from build123d import *

# Parameters (mm, degrees)
S01_BEARING_BARREL_R                             = 22
F_01_BEARING_BARREL_DEPTH                        = 21
F_02_TORQUE_ARM_1_DEPTH                          = 10
F_03_TORQUE_ARM_2_DEPTH                          = 10
F_04_TORQUE_ARM_3_DEPTH                          = 10
F_05_WHEEL_ARM_ROOT_TO_ROUNDED_ELBOW_DEPTH       = 10
F_06_LONG_DROPPED_WHEEL_ARM_DEPTH                = 10
F_07_BROAD_CAM_FOLLOWER_MOUNTING_LUG_DEPTH       = 10
F_08_START                                       = -1
S08_BEARING_THROUGH_RELIEF_R                     = 12
F_08_BEARING_THROUGH_RELIEF_DEPTH                = 23
F_09_START                                       = -0.1
S09_INBOARD_6001_SEAT_R                          = 14.1
F_09_INBOARD_6001_SEAT_DEPTH                     = 8.2
F_10_START                                       = 12.9
S10_OUTBOARD_6001_SEAT_R                         = 14.1
F_10_OUTBOARD_6001_SEAT_DEPTH                    = 8.2
F_11_START                                       = -1
S11_KEEPER_SCREWS_R                              = 1.7
F_11_KEEPER_SCREWS_DEPTH                         = 23
F_12_START                                       = -1
S12_TORQUE_PIN_RETAINING_STEMS_R                 = 3.25
F_12_TORQUE_PIN_RETAINING_STEMS_DEPTH            = 12
F_19_START                                       = -1
S19_THROUGH_BORE_FOR_STEEL_FOLLOWER_BU_R         = 5.1
F_19_THROUGH_BORE_FOR_STEEL_FOLLOWER_BUS_DEPTH   = 12
F_20_START                                       = -0.1
S20_FLUSH_SEAT_FOR_BUSH_FLANGE_R                 = 7.6
F_20_FLUSH_SEAT_FOR_BUSH_FLANGE_DEPTH            = 2.1
FLAT_MOTOR_MOUNTING_PAD_LAYOUT_R                 = 21
FLAT_MOTOR_MOUNTING_PAD_DEPTH                    = 10
R4_BLENDS_FROM_ARM_INTO_MOTOR_PAD_R              = 4
F_28_START                                       = 10.12
F_28_X_14_CLOSED_THROUGH_SLOT_FOR_MOTOR_OU_DEPTH = 10.24
SIX_START                                        = 10.12
SIX_CLEARANCE_HOLES_FROM_JOHNSON_MOT_2_R         = 1.65
SIX_CLEARANCE_HOLES_FROM_JOHNSON_MOTOR_F_DEPTH   = 10.24
F_01_START                                       = -0.1
S01_PRINTED_DRIVE_PIN_PILOT_BORES_R              = 4.1
F_01_PRINTED_DRIVE_PIN_PILOT_BORES_DEPTH         = 10.2
F_02_START                                       = -0.1
S02_FLUSH_SEATS_FOR_DRIVE_PIN_SHOULDER_R         = 5.4
F_02_FLUSH_SEATS_FOR_DRIVE_PIN_SHOULDERS_DEPTH   = 2.1


with BuildPart() as part:
    # S01 - Bearing barrel → 01 - Bearing barrel (new body)
    with BuildSketch(Plane.XY):
        with Locations(Location((0, 0, 0), (0, 0, 180))):
            Circle(S01_BEARING_BARREL_R)
    extrude(amount=F_01_BEARING_BARREL_DEPTH)

    # S02 - Torque arm 1 → 02 - Torque arm 1 (add)
    with BuildSketch(Plane.XY):
        with BuildLine():
            Line((0, 8), (36, 8))
            ThreePointArc((36, 8), (44, 0), (36, -8))
            Line((36, -8), (0, -8))
            ThreePointArc((0, -8), (-8, 0), (0, 8))
        make_face()
    extrude(amount=F_02_TORQUE_ARM_1_DEPTH)

    # S03 - Torque arm 2 → 03 - Torque arm 2 (add)
    with BuildSketch(Plane.XY):
        with BuildLine():
            Line((-6.92820323, -4), (-24.92820323, 27.176914536))
            ThreePointArc((-24.92820323, 27.176914536), (-22, 38.105117767), (-11.07179677, 35.176914536))
            Line((-11.07179677, 35.176914536), (6.92820323, 4))
            ThreePointArc((6.92820323, 4), (4, -6.92820323), (-6.92820323, -4))
        make_face()
    extrude(amount=F_03_TORQUE_ARM_2_DEPTH)

    # S04 - Torque arm 3 → 04 - Torque arm 3 (add)
    with BuildSketch(Plane.XY):
        with BuildLine():
            Line((6.92820323, -4), (-11.07179677, -35.176914536))
            ThreePointArc((-11.07179677, -35.176914536), (-22, -38.105117767), (-24.92820323, -27.176914536))
            Line((-24.92820323, -27.176914536), (-6.92820323, 4))
            ThreePointArc((-6.92820323, 4), (4, 6.92820323), (6.92820323, -4))
        make_face()
    extrude(amount=F_04_TORQUE_ARM_3_DEPTH)

    # S05 - Wheel arm root to rounded elbow → 05 - Wheel arm root to rounded elbow (add)
    with BuildSketch(Plane.XY):
        with BuildLine():
            Line((0.890943823, 12.969434032), (67.022341031, 8.426494092))
            ThreePointArc((67.022341031, 8.426494092), (79.10083124, -5.433883763), (65.240453385, -17.512373972))
            Line((65.240453385, -17.512373972), (-0.890943823, -12.969434032))
            ThreePointArc((-0.890943823, -12.969434032), (-12.969434032, 0.890943823), (0.890943823, 12.969434032))
        make_face()
    extrude(amount=F_05_WHEEL_ARM_ROOT_TO_ROUNDED_ELBOW_DEPTH)

    # S06 - Long dropped wheel arm → 06 - Long dropped wheel arm (add)
    with BuildSketch(Plane.XY):
        with BuildLine():
            Line((76.528125799, 1.449391376), (116.886494349, -68.572605409))
            ThreePointArc((116.886494349, -68.572605409), (112.482097074, -84.961665317), (96.093037167, -80.557268042))
            Line((96.093037167, -80.557268042), (55.734668617, -10.535271257))
            ThreePointArc((55.734668617, -10.535271257), (60.139065892, 5.853788651), (76.528125799, 1.449391376))
        make_face()
    extrude(amount=F_06_LONG_DROPPED_WHEEL_ARM_DEPTH)

    # S07 - Broad cam follower mounting lug → 07 - Broad cam follower mounting lug (add)
    with BuildSketch(Plane.XY):
        with BuildLine():
            Line((6.53566842, 10.064046815), (57.694573065, -23.158934321))
            ThreePointArc((57.694573065, -23.158934321), (61.22295146, -39.758649556), (44.623236224, -43.287027951))
            Line((44.623236224, -43.287027951), (-6.53566842, -10.064046815))
            ThreePointArc((-6.53566842, -10.064046815), (-10.064046815, 6.53566842), (6.53566842, 10.064046815))
        make_face()
    extrude(amount=F_07_BROAD_CAM_FOLLOWER_MOUNTING_LUG_DEPTH)

    # S08 - Bearing through relief → 08 - Bearing through relief (cut)
    with BuildSketch(Plane.XY.offset(F_08_START)):
        Circle(S08_BEARING_THROUGH_RELIEF_R)
    extrude(amount=F_08_BEARING_THROUGH_RELIEF_DEPTH, mode=Mode.SUBTRACT)

    # S09 - Inboard 6001 seat → 09 - Inboard 6001 seat (cut)
    with BuildSketch(Plane.XY.offset(F_09_START)):
        Circle(S09_INBOARD_6001_SEAT_R)
    extrude(amount=F_09_INBOARD_6001_SEAT_DEPTH, mode=Mode.SUBTRACT)

    # S10 - Outboard 6001 seat → 10 - Outboard 6001 seat (cut)
    with BuildSketch(Plane.XY.offset(F_10_START)):
        Circle(S10_OUTBOARD_6001_SEAT_R)
    extrude(amount=F_10_OUTBOARD_6001_SEAT_DEPTH, mode=Mode.SUBTRACT)

    # S11 - Keeper screws → 11 - Keeper screws (cut)
    with BuildSketch(Plane.XY.offset(F_11_START)):
        with Locations((0, 18.25)):
            Circle(S11_KEEPER_SCREWS_R)
        with Locations((-15.804963619, -9.125)):
            Circle(S11_KEEPER_SCREWS_R)
        with Locations((15.804963619, -9.125)):
            Circle(S11_KEEPER_SCREWS_R)
    extrude(amount=F_11_KEEPER_SCREWS_DEPTH, mode=Mode.SUBTRACT)

    # S12 - Torque pin retaining stems → 12 - Torque pin retaining stems (cut)
    with BuildSketch(Plane.XY.offset(F_12_START)):
        with Locations(Location((36, 0, 0), (0, 0, 180))):
            Circle(S12_TORQUE_PIN_RETAINING_STEMS_R)
        with Locations(Location((-18, 31.176914536, 0), (0, 0, 180))):
            Circle(S12_TORQUE_PIN_RETAINING_STEMS_R)
        with Locations(Location((-18, -31.176914536, 0), (0, 0, 180))):
            Circle(S12_TORQUE_PIN_RETAINING_STEMS_R)
    extrude(amount=F_12_TORQUE_PIN_RETAINING_STEMS_DEPTH, mode=Mode.SUBTRACT)

    # S19 - Through bore for steel follower bu → 19 - Through bore for steel follower bus (cut)
    with BuildSketch(Plane.XY.offset(F_19_START)):
        with Locations(Location((51.158904645, -33.222981136, 0), (0, 0, 180))):
            Circle(S19_THROUGH_BORE_FOR_STEEL_FOLLOWER_BU_R)
    extrude(amount=F_19_THROUGH_BORE_FOR_STEEL_FOLLOWER_BUS_DEPTH, mode=Mode.SUBTRACT)

    # S20 - Flush seat for bush flange → 20 - Flush seat for bush flange (cut)
    with BuildSketch(Plane.XY.offset(F_20_START)):
        with Locations((51.158904645, -33.222981136)):
            Circle(S20_FLUSH_SEAT_FOR_BUSH_FLANGE_R)
    extrude(amount=F_20_FLUSH_SEAT_FOR_BUSH_FLANGE_DEPTH, mode=Mode.SUBTRACT)

    # Flat motor mounting pad layout → Flat motor mounting pad (add)
    with BuildSketch(Plane.XY):
        with Locations((106.780015642, -75.748703358)):
            Circle(FLAT_MOTOR_MOUNTING_PAD_LAYOUT_R)
    extrude(amount=FLAT_MOTOR_MOUNTING_PAD_DEPTH)

    # R4 blends from arm into motor pad
    r4_blends_from_arm_into_motor_pad_edges = [part.edges().sort_by_distance(p)[0] for p in [
        (108.985808176, -54.864870393, 5),
        (87.956079001, -66.439599786, 5),
    ]]
    fillet(r4_blends_from_arm_into_motor_pad_edges, radius=R4_BLENDS_FROM_ARM_INTO_MOTOR_PAD_R)

    # Original round-ended output slot layout → 28 x 14 closed through slot for motor ou (cut)
    with BuildSketch(Plane.XY.offset(F_28_START)):
        with BuildLine():
            Line((96.668388671, -75.960835392), (106.567883608, -66.061340455))
            ThreePointArc((106.567883608, -66.061340455), (116.467378544, -66.061340455), (116.467378544, -75.960835392))
            Line((116.467378544, -75.960835392), (106.567883608, -85.860330328))
            ThreePointArc((106.567883608, -85.860330328), (96.668388671, -85.860330328), (96.668388671, -75.960835392))
        make_face()
    extrude(amount=-F_28_X_14_CLOSED_THROUGH_SLOT_FOR_MOTOR_OU_DEPTH, mode=Mode.SUBTRACT)

    # Six clearance holes from Johnson mot 2 → Six clearance holes from Johnson motor f (cut)
    with BuildSketch(Plane.XY.offset(SIX_START)):
        with Locations((92.035157904, -79.699576081)):
            Circle(SIX_CLEARANCE_HOLES_FROM_JOHNSON_MOT_2_R)
        with Locations((102.829142919, -90.493561096)):
            Circle(SIX_CLEARANCE_HOLES_FROM_JOHNSON_MOT_2_R)
        with Locations((117.574000657, -86.542688372)):
            Circle(SIX_CLEARANCE_HOLES_FROM_JOHNSON_MOT_2_R)
        with Locations((121.52487338, -71.797830634)):
            Circle(SIX_CLEARANCE_HOLES_FROM_JOHNSON_MOT_2_R)
        with Locations((110.730888366, -61.003845619)):
            Circle(SIX_CLEARANCE_HOLES_FROM_JOHNSON_MOT_2_R)
        with Locations((95.986030627, -64.954718343)):
            Circle(SIX_CLEARANCE_HOLES_FROM_JOHNSON_MOT_2_R)
    extrude(amount=-SIX_CLEARANCE_HOLES_FROM_JOHNSON_MOTOR_F_DEPTH, mode=Mode.SUBTRACT)

    # S01 - Printed drive pin pilot bores → 01 - Printed drive pin pilot bores (cut)
    with BuildSketch(Plane.XY.offset(F_01_START)):
        with Locations(Location((36, 0, 0), (0, 0, 180))):
            Circle(S01_PRINTED_DRIVE_PIN_PILOT_BORES_R)
        with Locations(Location((-18, 31.176914536, 0), (0, 0, 180))):
            Circle(S01_PRINTED_DRIVE_PIN_PILOT_BORES_R)
        with Locations(Location((-18, -31.176914536, 0), (0, 0, 180))):
            Circle(S01_PRINTED_DRIVE_PIN_PILOT_BORES_R)
    extrude(amount=F_01_PRINTED_DRIVE_PIN_PILOT_BORES_DEPTH, mode=Mode.SUBTRACT)

    # S02 - Flush seats for drive pin shoulder → 02 - Flush seats for drive pin shoulders (cut)
    with BuildSketch(Plane.XY.offset(F_02_START)):
        with Locations((36, 0)):
            Circle(S02_FLUSH_SEATS_FOR_DRIVE_PIN_SHOULDER_R)
        with Locations((-18, 31.176914536)):
            Circle(S02_FLUSH_SEATS_FOR_DRIVE_PIN_SHOULDER_R)
        with Locations((-18, -31.176914536)):
            Circle(S02_FLUSH_SEATS_FOR_DRIVE_PIN_SHOULDER_R)
    extrude(amount=F_02_FLUSH_SEATS_FOR_DRIVE_PIN_SHOULDERS_DEPTH, mode=Mode.SUBTRACT)


solid = part.part
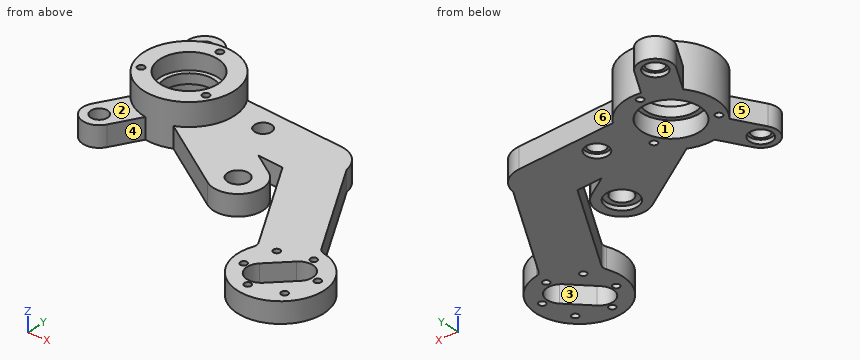
Input: part model. Units: mm. Frame: model coordinates. Face numbers are marked on the shaded views. A direction names the side the tool comes from. Round coordinates to 2 decimals unless told otherwise and drop trailing zeros. Order: outer loops, then holes, each group sorted by start corner. A loop starts at its lowest first (then second) coordinate and runs counter-clockwise, first axis right, second up.
1. Mould query, pull axis Y, two halves, no side actions, for the marked faces 4, 5 and 6. Classes: released by +Y, released by -Y, zero draft, split by the parting line, or undercut.
The answers:
face 4: released by -Y
face 5: undercut
face 6: released by +Y
2. Cut plane A-A, the plane x = 0. Output: boundary loops of the cut face in (y, z), then the cut area to 3 significant figures.
The answers:
outline: (-22, 0) - (-14.1, 0) - (-14.1, 8.1) - (-12, 8.1) - (-12, 12.9) - (-14.1, 12.9) - (-14.1, 21) - (-22, 21) - close; (12, 8.1) - (14.1, 8.1) - (14.1, 0) - (16.55, 0) - (16.55, 21) - (14.1, 21) - (14.1, 12.9) - (12, 12.9) - close; (19.95, 0) - (22, 0) - (22, 21) - (19.95, 21) - close
area: 281 mm2
3. Cut plane D-D, the plane y = 18.25. Output: boundary loops of the cut face in (x, z).
The answers:
outline: (-19.77, 0) - (-1.7, 0) - (-1.7, 21) - (-12.29, 21) - (-12.29, 10) - (-19.77, 10) - close; (1.7, 0) - (12.29, 0) - (12.29, 21) - (1.7, 21) - close
4. Set-up query: the marked faces 1, 2 and 3. Return all of +Z, -Z, +X, -X, +Y, -Y with unobstructed straight access to the full face (end or side cutting, diameter ignored); none if empty.
The answers:
face 1: -Z
face 2: +Z, -X, -Y
face 3: +Z, -Z
5. Pin query (flat end, axial travel): P1, Ø4.5, axis at x = 117.57, y = -86.54, coming from the -Z side; P2, Ø5, axis at y = -68, z = 5, coming from the +X side; P3, Ø2, axis at x = 15.8, y = -9.12, coming from the +Z side; P4, Ø5, axis at y = -54, z = 9.5, coming from the -X side. Return the tip coordinate at first contact, or that it passes through.
The answers:
P1: stops at z = 0
P2: stops at x = 127.11
P3: passes through
P4: stops at x = 79.35
6. Cut plane B-B, the plane y = 0. Output: boundary loops of the cut face in (x, z), then the cut area to 3 significant figures.
The answers:
outline: (-22, 0) - (-14.1, 0) - (-14.1, 8.1) - (-12, 8.1) - (-12, 12.9) - (-14.1, 12.9) - (-14.1, 21) - (-22, 21) - close; (12, 8.1) - (14.1, 8.1) - (14.1, 0) - (30.6, 0) - (30.6, 2) - (31.9, 2) - (31.9, 10) - (22, 10) - (22, 21) - (14.1, 21) - (14.1, 12.9) - (12, 12.9) - close; (40.1, 2) - (41.4, 2) - (41.4, 0) - (78.31, 0) - (78.31, 10) - (40.1, 10) - close
area: 828 mm2
7. Material intervals for line 1 (Y direction, x = 0, z = 16); line 2 (Y direction, x = 55.5, z = 6); line 3 (Z direction, x = 83, y = -41.5), sorted ascending.
The answers:
line 1: y = -22 to -14.1, 14.1 to 16.55, 19.95 to 22
line 2: y = -44.41 to -35.9, -30.55 to -21.73, -16.84 to 9.22
line 3: z = 0 to 10
8. Cut plane C-C, the plane x = 36. Output: boundary loops of the cut face in (y, z), then the cut area to 3 significant figures.
The answers:
outline: (-37.69, 0) - (-5.4, 0) - (-5.4, 2) - (-4.1, 2) - (-4.1, 10) - (-37.69, 10) - close; (4.1, 2) - (5.4, 2) - (5.4, 0) - (10.56, 0) - (10.56, 10) - (4.1, 10) - close
area: 395 mm2
